```python
from build123d import *

# Parameters (mm, degrees)
F0_W     = 60
F0_H     = 40
F0_R     = 3.25
F1_DEPTH = 5
F0_R_2   = 1.65
F2_DEPTH = 3


with BuildPart() as f1:
    # F0 (on Top) → F1 (new body)
    with BuildSketch(Plane.XY):
        Rectangle(F0_W, F0_H)
        with Locations((-15.25, 10)):
            Circle(F0_R, mode=Mode.SUBTRACT)
        with Locations((15.25, 10)):
            Circle(F0_R, mode=Mode.SUBTRACT)
    extrude(amount=F1_DEPTH)

    # F0 (on Top) → F2 (join)
    with BuildSketch(Plane.XY):
        with Locations((15.25, 10)):
            Circle(F0_R)
        with Locations((15.25, 10)):
            Circle(F0_R_2, mode=Mode.SUBTRACT)
        with Locations((-15.25, 10)):
            Circle(F0_R)
        with Locations((-15.25, 10)):
            Circle(F0_R_2, mode=Mode.SUBTRACT)
    extrude(amount=F2_DEPTH)


solid = f1.part
```
Check sheet for the modelled part. Datum: model origin and axes. Units: mm. A direction names the side the tool comes from. Round coordinates to 2 decimals unless told otherwise and drop trailing zeros. Write each loop counter-clockwise with the first axis right and the second up, starting at its lowest first coordinate (ties: lowest second). Pieces come first, ordered by that corner, then holes. Notation, with made-up numbers: M -13,55 L 13,55 A13 ccw 13,70 Z; hole C 29,49 d9. An arc over 180 degrees is marked long. Write item = value, one per line. Start each with the question number.
1. Gauge pin test, flat ends, axial feed: pin 1 (2 mm diameter, centred on x = -8, y = -15.5, fed in from -Z); pin 2 (3 mm diameter, centred on x = 14.5, y = 11.5, fed in from +Z); pin 3 (3 mm diameter, centred on x = -15.25, y = 10, fed in from +Z). Record the tip position at first contact, or that the pin passes through.
2. Section check A-A, the plane x = -15.25. Record the cut outline in (y, z).
3. Tool access check on faces 1 (the cylindrical face through (14.827, 13.222, 3.986)), 2 (the flat face through (30, 0, 2)). Record the directions out of +Z, -Z, +X, -X, +Y, -Y that give a thin tool (end or side, any length) a straight path to the whole face; none if there is none.
4. Section check B-B, the plane y = 10. Record the cut outline in (x, z).
5. Release check for a two-part mould opening along X. For faces 3 (the flat face through (0, 20, 2)), 4 (the cylindrical face through (16.774, 9.368, 1.479)), 5 (the flat face through (-30, 0, 2)) record: pulls with the +X half, pulls with the -X half, needs draft (parallel to the pull), parting line crosses it, or undercut.
6. Scan lines: line 1 (Y direction, x = -15.25, z = 1.25); line 2 (Y direction, x = -15.25, z = 3.45); line 3 (X direction, y = 11, z = 4.5). Record each from-to range of solid material in increasing order. Write a range as [from, to].
Results found:
q1.pin_1 = 0
q1.pin_2 = 3
q1.pin_3 = through
q2.outline = M -20,0 L 8.35,0 L 8.35,3 L 6.75,3 L 6.75,5 L -20,5 Z; M 11.65,0 L 20,0 L 20,5 L 13.25,5 L 13.25,3 L 11.65,3 Z
q3.face_1 = +Z
q3.face_2 = +Z, -Z, +X, +Y, -Y
q4.outline = M -30,0 L -16.9,0 L -16.9,3 L -18.5,3 L -18.5,5 L -30,5 Z; M -13.6,0 L 13.6,0 L 13.6,3 L 12,3 L 12,5 L -12,5 L -12,3 L -13.6,3 Z; M 16.9,0 L 30,0 L 30,5 L 18.5,5 L 18.5,3 L 16.9,3 Z
q5.face_3 = needs draft
q5.face_4 = undercut
q5.face_5 = pulls with the -X half
q6.line_1 = [-20, 8.35], [11.65, 20]
q6.line_2 = [-20, 6.75], [13.25, 20]
q6.line_3 = [-30, -18.34], [-12.16, 12.16], [18.34, 30]
